Read the model definition and answer for the solid it produces. Units are mm, in the model's axes. A direction names the side the tool comes from. Give positions to 0.01 mm unless a question says otherwise; leave off trailing zeros. Order: outer loops, then holes, each group sorted by start corner. A loop starts at its lowest first (then second) coordinate and runs counter-clockwise, first axis right, second up. Notation, with made-up numbers: (57.5, -20) - (63.5, -20) arc R18 ccw to (63.5, 3) - close; hole circle Ø7 at (84, 83.5). An arc over 180 degrees is marked (long way). Write item = value, one per line.
```python
from build123d import *

# Parameters (mm, degrees)
F0_R     = 1
F0_R_2   = 3
F0_R_3   = 1.5
F1_DEPTH = 3


with BuildPart() as f1:
    # F0 (on Front) → F1 (new body)
    with BuildSketch(Plane.XZ):
        with BuildLine():
            Line((-23.863873, -18.387415), (-3.880417, -18.387415))
            ThreePointArc((-3.880417, -18.387415), (-0.814886, -19.437413), (0.963125, -22.146408))
            Line((0.963125, -22.146408), (10.337516, -58.733814))
            ThreePointArc((10.337516, -58.733814), (21.289706, -65.218376), (27.774267, -54.266186))
            Line((27.774267, -54.266186), (19.277183, -21.102826))
            ThreePointArc((19.277183, -21.102826), (19.715388, -17.496865), (22.478727, -15.139124))
            Line((22.478727, -15.139124), (34.22563, -11.054934))
            ThreePointArc((34.22563, -11.054934), (36.658555, -9.229653), (37.583633, -6.332239))
            Line((37.583633, -6.332239), (37.583633, -5.887415))
            Line((37.583633, -5.887415), (37.583633, 5.887415))
            Line((37.583633, 5.887415), (37.583633, 6.332239))
            ThreePointArc((37.583633, 6.332239), (36.658555, 9.229653), (34.22563, 11.054934))
            Line((34.22563, 11.054934), (22.478727, 15.139124))
            ThreePointArc((22.478727, 15.139124), (19.715388, 17.496865), (19.277183, 21.102826))
            Line((19.277183, 21.102826), (27.774267, 54.266186))
            ThreePointArc((27.774267, 54.266186), (21.289706, 65.218376), (10.337516, 58.733814))
            Line((10.337516, 58.733814), (0.963125, 22.146408))
            ThreePointArc((0.963125, 22.146408), (-0.814886, 19.437413), (-3.880417, 18.387415))
            Line((-3.880417, 18.387415), (-23.636704, 18.387415))
            ThreePointArc((-23.636704, 18.387415), (-25.616733, 18.796175), (-27.273019, 19.955621))
            Line((-27.273019, 19.955621), (-51.547948, 45.67723))
            ThreePointArc((-51.547948, 45.67723), (-64.326865, 45.991752), (-64.530968, 33.210594))
            Line((-64.530968, 33.210594), (-45.747828, 13.984717))
            ThreePointArc((-45.747828, 13.984717), (-44.061446, 11.412506), (-43.470186, 8.394134))
            Line((-43.470186, 8.394134), (-43.470186, -8.038917))
            ThreePointArc((-43.470186, -8.038917), (-44.047755, -11.023464), (-45.697065, -13.577065))
            Line((-45.697065, -13.577065), (-64.588075, -33.269584))
            ThreePointArc((-64.588075, -33.269584), (-64.281862, -46.034668), (-51.51901, -45.646423))
            Line((-51.51901, -45.646423), (-27.516265, -19.972736))
            ThreePointArc((-27.516265, -19.972736), (-25.854677, -18.800837), (-23.863873, -18.387415))
        make_face()
        with Locations((-58.093314, -44)):
            Circle(F0_R, mode=Mode.SUBTRACT)
        with Locations((-58.093314, -39.5)):
            Circle(F0_R_2, mode=Mode.SUBTRACT)
        with Locations((-58.093314, -35)):
            Circle(F0_R, mode=Mode.SUBTRACT)
        with BuildLine():
            ThreePointArc((-36.083633, -8), (-38.646085, -9.058865), (-37.578558, -6.500009))
            ThreePointArc((-37.578558, -6.500009), (-36.52118, -6.941135), (-36.083633, -8))
        make_face(mode=Mode.SUBTRACT)
        with Locations((-22.583633, -15.25)):
            Circle(F0_R_3, mode=Mode.SUBTRACT)
        with Locations((16.592031, -60.265553)):
            Circle(F0_R, mode=Mode.SUBTRACT)
        with Locations((19.055892, -56.5)):
            Circle(F0_R_2, mode=Mode.SUBTRACT)
        with Locations((21.446564, -52.687562)):
            Circle(F0_R, mode=Mode.SUBTRACT)
        with Locations((7.916367, -15.25)):
            Circle(F0_R_3, mode=Mode.SUBTRACT)
        with Locations((32.916367, -8.5)):
            Circle(F0_R, mode=Mode.SUBTRACT)
        with BuildLine():
            ThreePointArc((-37.55657, 5.322031), (-37.515348, 5.367937), (-37.473773, 5.413524))
            Line((-37.473773, 5.413524), (-37.55657, 5.321561))
            Line((-37.55657, 5.321561), (-37.583633, 5.291503))
            ThreePointArc((-37.583633, 5.291503), (-37.570121, 5.306784), (-37.55657, 5.322031))
        make_face(mode=Mode.SUBTRACT)
        with BuildLine():
            ThreePointArc((-36.05657, 8), (-36.49591, 6.93934), (-37.55657, 6.5))
            ThreePointArc((-37.55657, 6.5), (-38.61723, 9.06066), (-36.05657, 8))
        make_face(mode=Mode.SUBTRACT)
        with Locations((-22.583633, 15.25)):
            Circle(F0_R_3, mode=Mode.SUBTRACT)
        with Locations((-58.247652, 35.002647)):
            Circle(F0_R, mode=Mode.SUBTRACT)
        with Locations((-58.093314, 39.5)):
            Circle(F0_R_2, mode=Mode.SUBTRACT)
        with Locations((-58.015386, 43.999325)):
            Circle(F0_R, mode=Mode.SUBTRACT)
        with Locations((7.916367, 15.25)):
            Circle(F0_R_3, mode=Mode.SUBTRACT)
        with Locations((32.916367, 8.5)):
            Circle(F0_R, mode=Mode.SUBTRACT)
        with Locations((19.055892, 56.5)):
            Circle(F0_R_2, mode=Mode.SUBTRACT)
        with Locations((22.380625, 53.467484)):
            Circle(F0_R, mode=Mode.SUBTRACT)
        with Locations((15.694703, 59.492058)):
            Circle(F0_R, mode=Mode.SUBTRACT)
    extrude(amount=F1_DEPTH)


solid = f1.part
```
1. Straight lines are drawn through the part: L1, parallel to X at y = -2.35, z = -37.5; L2, parallel to Z at x = -22, y = -0.7; L3, parallel to X at y = -0.8, z = -42 (3 decimals). For each, find the intervals that lie inside material, in ascending order. Write a range as [from, to].
Recorded:
L1 = [-66.87, -60.33], [-55.86, -43.9], [4.9, 23.48]
L2 = [-18.39, -16.63], [-13.87, 13.87], [16.63, 18.39]
L3 = [-66.739, -59.752], [-56.435, -48.11], [6.05, 24.631]
2. Section A-A (z = 39.5) is taken. Determine the outline of the cut face in (x, y).
Recorded:
outline = (-67.09, -3) - (-61.09, -3) - (-61.09, 0) - (-67.09, 0) - close; (-55.09, -3) - (-45.72, -3) - (-45.72, 0) - (-55.09, 0) - close; (5.41, -3) - (23.99, -3) - (23.99, 0) - (5.41, 0) - close
3. Section C-C (z = 56.5) is taken. Determine the outline of the cut face in (x, y), and give its area (3 significant figures).
Recorded:
outline = (9.77, -3) - (16.06, -3) - (16.06, 0) - (9.77, 0) - close; (22.06, -3) - (28.06, -3) - (28.06, 0) - (22.06, 0) - close
area = 36.9 mm^2
4. Section B-B (x = -49) is taken. Determine the outline of the cut face in (y, z).
Recorded:
outline = (-3, -42.95) - (0, -42.95) - (0, -17.02) - (-3, -17.02) - close; (-3, 17.31) - (0, 17.31) - (0, 42.98) - (-3, 42.98) - close
5. For faces 1 (the face through (-0.85, -1.48, -19.41)), 2 (the face through (19.691, -1.479, -17.543)), 3 (the face through (18.665, -1.479, 59.474)), 4 (the face through (5.716, -1.479, 40.696)), 5 (the face through (-55.01, -1.479, -23.285)), determine the directions among +Z, -Z, +X, -X, +Y, -Y from which every point of the face is accessible in a straight line to the end or side of a thin tool.
Recorded:
face_1 = -Z, +Y, -Y
face_2 = +X, +Y, -Y
face_3 = +Y, -Y
face_4 = +Z, +Y, -Y
face_5 = -X, +Y, -Y
6. Flat-ended cylindrical pins translate along their axes: pin 1 (2.5 mm diameter, centred on x = -37.56, z = 8, fed in from +Y); pin 2 (3.5 mm diameter, centred on x = -37.58, z = -8, fed in from -Y); pin 3 (0.9 mm diameter, centred on x = -17, y = -2, fed in from -Z); pin 4 (0.9 mm diameter, centred on x = -12.5, y = -1.5, fed in from +Z). Find the tip coordinate at first contact, or state that the pin passes through.
Recorded:
pin_1 = through
pin_2 = -3
pin_3 = -18.39
pin_4 = 18.39
7. Determine the mould class of faces 6 (the face through (-15, -3, 1)), 7 (the face through (-0.779, -1.479, 19.466)), 8 (the face through (-25.88, -1.48, -18.81)), 9 (the face through (9.347, -1.479, 15.701)) for opening direction Z: +Z half, -Z half, draft (parallel to the pull), parting line (faces both ways), or undercut.
Recorded:
face_6 = draft
face_7 = +Z half
face_8 = -Z half
face_9 = undercut
